```python
from build123d import *

# Parameters (mm, degrees)
SKETCH_W      = 12.1
SKETCH_H      = 14.1
PAD_DEPTH     = 3
SKETCH001_W   = 12.1
SKETCH001_H   = 14.1
SKETCH001_W_2 = 10.5
SKETCH001_H_2 = 12.5
PAD001_DEPTH  = 4
SKETCH002_R   = 4
POCKET_DEPTH  = 5


with BuildPart() as part:
    # Sketch → Pad (new body)
    with BuildSketch(Plane.XY):
        Rectangle(SKETCH_W, SKETCH_H)
    extrude(amount=PAD_DEPTH)

    # Sketch001 (on Face6 of Pad) → Pad001 (join)
    with BuildSketch(Plane.XY.offset(3)):
        Rectangle(SKETCH001_W, SKETCH001_H)
        Rectangle(SKETCH001_W_2, SKETCH001_H_2, mode=Mode.SUBTRACT)
    extrude(amount=PAD001_DEPTH)

    # Sketch002 (on Face6 of Pad001) → Pocket (cut)
    with BuildSketch(Plane.XY.offset(3)):
        Circle(SKETCH002_R)
    extrude(amount=-POCKET_DEPTH, mode=Mode.SUBTRACT)


solid = part.part
```
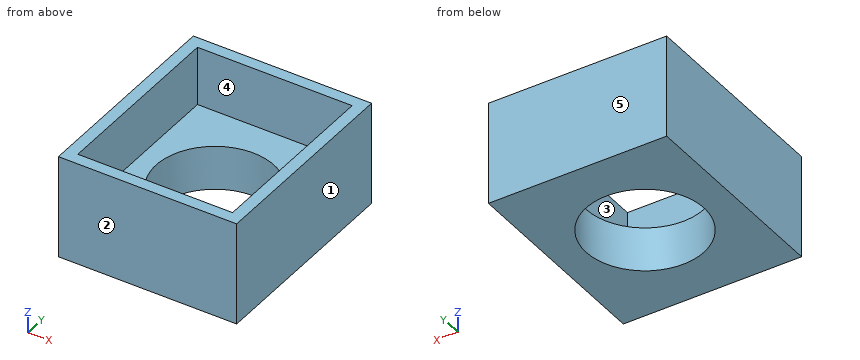
The listing builds one solid part. Answer for the finished solid, in the listing's coordinates (mm). Face numbers are marked on the shaded views. A direction names the side the tool comes from. Give positions to 0.01 mm unless a question says otherwise; leave off trailing zeros. Order: outer loops, then holes, each group sorted by start corner. A loop starts at its lowest first (then second) coordinate and runs counter-clockwise, first axis right, second up. Notation, with made-up numbers: (-16, 14) -> (-1, 14) arc R19 ccw to (-1, 30) -> close; hole circle Ø2 at (52.25, -36.5). An arc over 180 degrees is marked (long way). Answer as a JSON object with one key per item and string values. Group by question number.
Item 1: Consider L1, parallel to Y at x = 0, z = 1.75; L2, parallel to X at y = 6, z = 6.25; L3, parallel to Y at x = -2.25, z = 5.75. Determine where each line is inside the solid, lowest interval first. Write a range as from..to.
Item 2: Determine the mould class of the marked faces 1, 2 and 3 for opening direction Y: pulls with the +Y half, pulls with the -Y half, needs draft (parallel to the pull), parting line crosses it, or undercut.
Item 3: The part is cut by section D-D on y = 5.5. Write down the section's boundary in (x, z).
Item 4: The part is cut by section B-B on z = 6. Write down the section's boundary in (x, y).
Item 5: A tool of negligible diameter and unlimited length cuts with its end or side. For the marked faces 4 and 5, from which of +Z, -Z, +X, -X, +Y, -Y can it reach the whole face along a straight path? Write none if from no direction.
Item 6: The part is cut by section A-A on y = 0. Write down the section's boundary in (x, z).
Item 7: A flat-ended cylindrical pin translates along its axis: pin 1 (3 mm diameter, centred on x = 1.5, y = 2.5, fed in from +Z). Find the tip coordinate at first contact, or state that the pin passes through.
Item 8: The part is cut by section C-C on x = 0. Write down the section's boundary in (y, z), and give its area (3 significant figures).
Result set:
{
 "1": {"L1": "-7.05..-4, 4..7.05", "L2": "-6.05..-5.25, 5.25..6.05", "L3": "-7.05..-6.25, 6.25..7.05"},
 "2": {"face 1": "needs draft", "face 2": "pulls with the -Y half", "face 3": "undercut"},
 "3": {"outline": "(-6.05, 0) -> (6.05, 0) -> (6.05, 7) -> (5.25, 7) -> (5.25, 3) -> (-5.25, 3) -> (-5.25, 7) -> (-6.05, 7) -> close"},
 "4": {"outline": "(-6.05, -7.05) -> (6.05, -7.05) -> (6.05, 7.05) -> (-6.05, 7.05) -> close; hole (-5.25, -6.25) -> (5.25, -6.25) -> (5.25, 6.25) -> (-5.25, 6.25) -> close"},
 "5": {"face 4": "+Z", "face 5": "+Z, -Z, +X, -X, +Y"},
 "6": {"outline": "(-6.05, 0) -> (-4, 0) -> (-4, 3) -> (-5.25, 3) -> (-5.25, 7) -> (-6.05, 7) -> close; (4, 0) -> (6.05, 0) -> (6.05, 7) -> (5.25, 7) -> (5.25, 3) -> (4, 3) -> close"},
 "7": {"pin 1": "z = 3"},
 "8": {"outline": "(-7.05, 0) -> (-4, 0) -> (-4, 3) -> (-6.25, 3) -> (-6.25, 7) -> (-7.05, 7) -> close; (4, 0) -> (7.05, 0) -> (7.05, 7) -> (6.25, 7) -> (6.25, 3) -> (4, 3) -> close", "area": "24.7 mm²"}
}
